The listing builds one solid part. Answer for the finished solid, in the listing's coordinates (mm). A direction names the side the tool comes from. Round coordinates to 2 decimals unless told otherwise and drop trailing zeros. Write each loop counter-clockwise with the first axis right and the second up, starting at its lowest first coordinate (ties: lowest second). Pieces come first, ordered by that corner, then holes.
Item 1: A tool of negligible diameter and unlimited length cuts with its end or side. For faces 1 (the face through (-25.592, -9.601, 7.395)), 2 (the face through (-30, -9, 15)), from which of +Z, -Z, +X, -X, +Y, -Y can it reach the whole face along a straight path? Write none if from no direction.
Item 2: Find section D-D on x = -32. Give the number of separate pieces and of enclosed holes in the cut face, then the cut area to 3 significant figures.
Item 3: Find section C-C on z = 15.75. Give the vertices of the cut face in (x, y), then the cut area to 3 significant figures.
Item 4: Find the intervals of material crossed by probe 1 along Y at (x, z) = (-27.5, 9.5); probe 2 along X at (y, z) = (9, 6.5); probe 3 along Y at (x, z) = (-30.5, 6.5), in increasing order.
Item 5: Each of these flat-tipped pins is pushed along its axis until it touches: pin 1 (3 mm diameter, centred on x = -28, z = 18, fed in from -Y); pin 2 (1.5 mm diameter, centred on x = -27, y = -7.5, fed in from +Z); pin 3 (2 mm diameter, centred on x = -28.5, z = 17.5, fed in from +Y). Where does it stop, or does it pass through?
Item 6: Find section B-B on z = 9.25. Give the vertices of the cut face in (x, y).
Item 7: Find section A-A on y = 9. Give the vertices of the cut face in (x, z), then the cut area to 3 significant figures.
Item 8: For a pull along Y with two mould halves and no side action, classify faces 3 (the face through (-30, 9, 15)), 4 (the face through (-25.592, 8.399, 7.395)), 5 (the face through (-30, -5, 17)), 6 (the face through (-30, 5, 17)) as +Y half, -Y half, draft (parallel to the pull), parting line (faces both ways), or undercut.
Autodesk Inventor part; units mm, degrees
ref_plane "Work Plane2" through (-37, -13, 19) normal (0, 0, -1) x (0, 1, 0)
ref_plane "YZ Plane" through (0, 0, 0) normal (1, 0, 0) x (0, 1, 0)
ref_plane "XZ Plane" through (0, 0, 0) normal (0, 1, 0) x (-1, 0, 0)
ref_plane "Work Plane1" through (0, 0, 0) normal (0, 0, 1) x (1, 0, 0)
sketch "Sketch1" plane through (0, 0, 0) normal (0, 0, 1) x (1, 0, 0)
  circle A0 centre (-27.5, 9) radius 2
  circle A1 centre (-27.5, -9) radius 2
  circle A2 centre (-30.5, 0) radius 2.5
  line L0 (-25, 13) -> (-25, -12.5061)
  line L1 (-35, -13) -> (-35, 13)
  line L2 (-25, -12.5061) -> (-25, -13)
  line L3 (-25, -13) -> (-35, -13)
  line L4 (-35, 13) -> (-25, 13)
  arc A3 (-2.9901, -1.4163) -> (-18.371, -4.3253) centre (-12.371, 6.067) ccw construction
  line L5 (-35, -13) -> (-35, 13) construction
  line L6 (-60.2, 0) -> (60.2, 0) construction
  point P0 (0, 0)
  dimension "d31" = 2.5
  dimension "d37" = 26
ref_plane "Work Plane2" through (-37, -13, 19) normal (0, 0, -1) x (0, 1, 0)
extrude "Extrusion1" add sketch "Sketch1" along normal up to surface (19 mm away)
ref_plane "Work Plane3" through (-0.8627, 0, 12) normal (0, 0, 1) x (1, 0, 0)
sketch "Sketch4" plane through (-0.8627, 0, 12) normal (0, 0, 1) x (1, 0, 0)
  circle A0 centre (-29.6373, 0) radius 2.5 construction
  circle A1 centre (-26.6373, -9) radius 2 construction
  circle A2 centre (-26.6373, 9) radius 2 construction
  line L0 (-34.1373, -13) -> (-24.1373, -13) construction
  line L1 (-24.1373, -13) -> (-24.1373, 13) construction
  line L2 (-24.1373, 13) -> (-34.1373, 13) construction
  line L3 (-34.1373, 13) -> (-34.1373, -13) construction
  line L4 (-24.1373, 13) -> (-24.1373, -13) construction
  line L5 (-24.1373, -3.2174) -> (-34.1373, -11.6084) construction
  line L6 (-34.1373, -13) -> (-34.1373, 13) construction
  line L7 (-24.1373, -1.2593) -> (-34.1373, -9.6503) construction
  line L8 (-24.1373, 0.6988) -> (-34.1373, -7.6922) construction
  line L9 (-23.1842, -0.4595) -> (-35.6373, -10.9089)
  point P0 (0.8627, 0)
  dimension "d7" = 130
  dimension "d8" = 1.5
  dimension "d9" = 1.5
  dimension "d10" = 0.5
  dimension "d13" = 1.5
ref_plane "Work Plane6" through (-35, -7.6922, 12) normal (-0.766, -0.6428, 0) x (0.6428, -0.766, 0)
sketch "Sketch7" plane through (-35, -7.6922, 12) normal (-0.766, -0.6428, 0) x (0.6428, -0.766, 0)
  point P0 (16.605, -12)
  point P1 (1.5, 0)
  point P2 (1.5, 0)
  point P3 (1.5, 0)
hole "Hole1" at (-34.0358, -8.8412, 12) direction (0.766, 0.6428, 0) diameter 2.459 end through all
hole "Hole2" at (-34.0358, -8.8412, 12) direction (-0.766, -0.6428, 0) diameter 2.459 end through all
sketch "Sketch9" plane through (-35, -13, 0) normal (-1, 0, 0) x (0, 0, 1)
  line L0 (19, 26) -> (15, 26)
  line L1 (15, 26) -> (15, 18)
  line L2 (15, 18) -> (19, 18)
  line L3 (19, 18) -> (19, 26)
  line L4 (19, 0) -> (15, 0)
  line L5 (15, 0) -> (15, 8)
  line L6 (15, 8) -> (19, 8)
  line L7 (19, 8) -> (19, 0)
  point P0 (0, 13)
  dimension "d32" = 4
  dimension "d33" = 8
extrude "Extrusion2" cut sketch "Sketch9" against normal up to surface (10 mm away)
fillet "Fillet1" radius 2 4 edges at (-25, 13, 7.5) (-35, 13, 7.5) (-35, -13, 7.5) (-25, -13, 7.5)
Check values:
1. face 1: +Z, -Z
1. face 2: +Z, +X, -X, -Y
2. separate pieces: 2
2. enclosed holes: 1
2. area: 348 mm2
3. outline: (-35, -5) - (-25, -5) - (-25, 5) - (-35, 5) - close; hole circle Ø5 at (-30.5, 0)
3. area: 80.4 mm2
4. probe 1: y = -13 to -11, -7 to 7, 11 to 13
4. probe 2: x = -35 to -29.5, -25.5 to -25
4. probe 3: y = -13 to -2.5, 2.5 to 13
5. pin 1: stops at y = -5
5. pin 2: stops at z = 15
5. pin 3: stops at y = 5
6. outline: (-35, -11) arc R2 ccw to (-33, -13) - (-27, -13) arc R2 ccw to (-25, -11) - (-25, 11) arc R2 ccw to (-27, 13) - (-33, 13) arc R2 ccw to (-35, 11) - close; hole circle Ø5 at (-30.5, 0); hole circle Ø4 at (-27.5, -9); hole circle Ø4 at (-27.5, 9)
7. outline: (-35, 0) - (-29.5, 0) - (-29.5, 15) - (-35, 15) - close; (-25.5, 0) - (-25, 0) - (-25, 15) - (-25.5, 15) - close
7. area: 90.0 mm2
8. face 3: draft
8. face 4: undercut
8. face 5: -Y half
8. face 6: +Y half
